Check sheet for the drawn part. Datum: minimum x, y, z corner. Units: mm. A direction names the side the tool comes from. Give positions to 0.01 mm unless a question says otherwise; leave off trailing zeros. Write each loop counter-clockwise with the first axis right and the second up, starting at its lowest first coordinate (ties: lowest second). Pieces come first, ordered by that corner, then holes. Notation, with made-up numbers: (-7, -9.5) - (15, -9.5) arc R24 ccw to (15, 8.5) - close; hole circle Ø3 at (64.25, 38.25). An arc over 180 degrees is marked (long way). Answer as a JSON object with one key per item and string values. Group by question number.
Item 1: Scan lines: line 1 along Y through (x, z) = (26.91, 38); line 2 along X through (y, z) = (26, 38); line 3 along Z through (x, y) = (48, 32). Record each from-to range of solid material in increasing order. Write a range as [from, to].
Item 2: Draft check along X on the marked faces 4, 5, 6 and 7. Enter one of: +X half, -X half, draft (parallel to the pull), parting line (faces both ways), or undercut.
Item 3: Sectioned sample at A-A, the plane y = 26.91. Record the boundary of the cut face in (x, z) (3 decimals), and give its area (3 significant figures).
Item 4: Tool access check on the marked faces 1, 2 and 3. Record the directions out of +Z, -Z, +X, -X, +Y, -Y that give a thin tool (end or side, any length) a straight path to the whole face; none if there is none.
Item 5: Sectioned sample at D-D, the plane y = 5.46. Record the boundary of the cut face in (x, z) (3 decimals), and give its area (3 significant figures).
Item 6: Sectioned sample at C-C, the plane z = 39.5. Record the boundary of the cut face in (x, y), and give its area (3 significant figures).
Item 7: Go/stop test with flat-tipped pins: pin 1 (4.5 mm diameter, centred on x = 26.91, y = 48.36, fed in from -Z); pin 2 (3 mm diameter, centred on y = 28, z = 29, fed in from +X) (3 decimals); pin 3 (7 mm diameter, centred on x = 5.46, y = 26.91, fed in from +Z); pin 4 (8.5 mm diameter, centred on x = 5.46, y = 26.91, fed in from -Z). Record where each tip stops, or that it passes through.
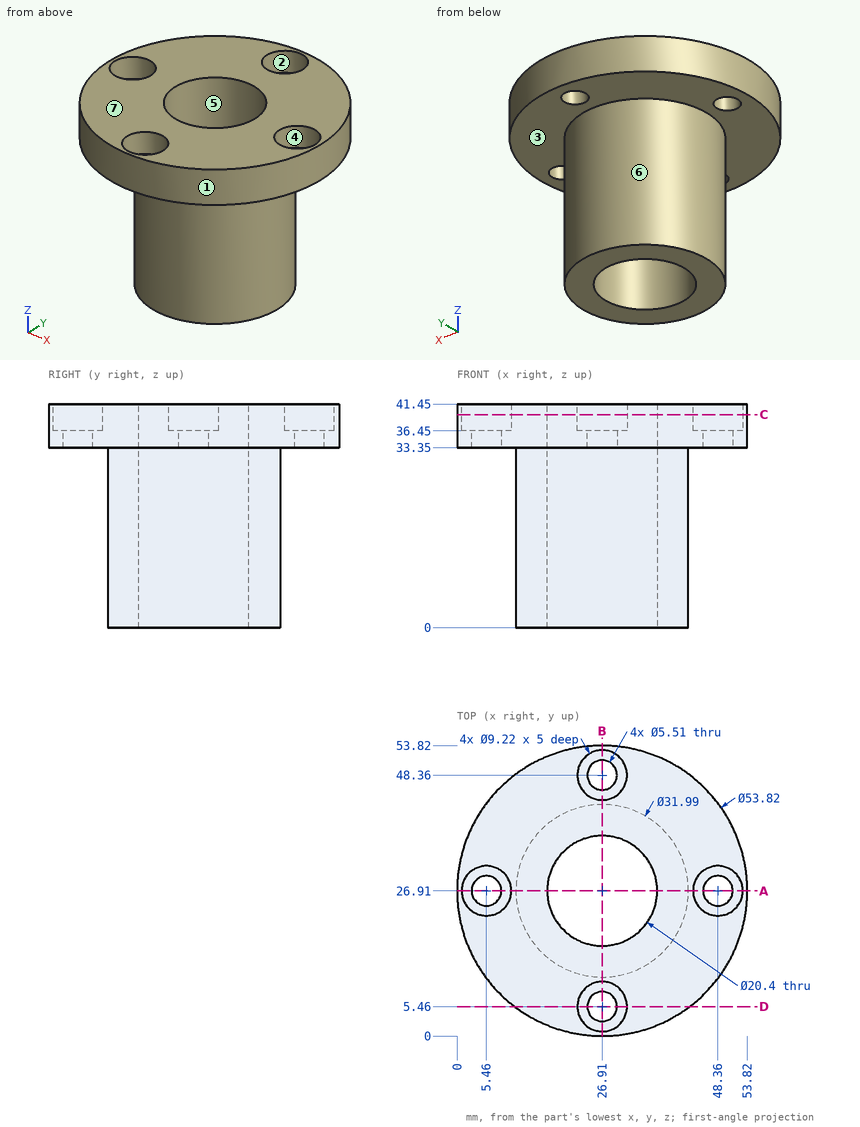
Geometry check:
{
 "1": {"line 1": "[0, 0.85], [10.07, 16.71], [37.11, 43.75], [52.97, 53.82]", "line 2": "[0.02, 0.94], [9.98, 16.75], [37.07, 43.84], [52.88, 53.8]", "line 3": "[33.35, 41.45]"},
 "2": {"face 4": "undercut", "face 5": "undercut", "face 6": "parting line", "face 7": "draft"},
 "3": {"outline": "(0, 33.35) - (2.705, 33.35) - (2.705, 36.45) - (0.85, 36.45) - (0.85, 41.45) - (0, 41.45) - close; (8.215, 33.35) - (10.915, 33.35) - (10.915, 0) - (16.71, 0) - (16.71, 41.45) - (10.07, 41.45) - (10.07, 36.45) - (8.215, 36.45) - close; (37.11, 0) - (42.905, 0) - (42.905, 33.35) - (45.605, 33.35) - (45.605, 36.45) - (43.75, 36.45) - (43.75, 41.45) - (37.11, 41.45) - close; (51.115, 33.35) - (53.82, 33.35) - (53.82, 41.45) - (52.97, 41.45) - (52.97, 36.45) - (51.115, 36.45) - close", "area": "531 mm^2"},
 "4": {"face 1": "+Z, -Z", "face 2": "+Z", "face 3": "-Z"},
 "5": {"outline": "(10.661, 33.35) - (24.155, 33.35) - (24.155, 36.45) - (22.3, 36.45) - (22.3, 41.45) - (10.661, 41.45) - close; (29.665, 33.35) - (43.159, 33.35) - (43.159, 41.45) - (31.52, 41.45) - (31.52, 36.45) - (29.665, 36.45) - close", "area": "200 mm^2"},
 "6": {"outline": "circle Ø53.82 at (26.91, 26.91); hole circle Ø9.22 at (5.46, 26.91); hole circle Ø20.4 at (26.91, 26.91); hole circle Ø9.22 at (26.91, 5.46); hole circle Ø9.22 at (26.91, 48.36); hole circle Ø9.22 at (48.36, 26.91)", "area": "1,680 mm^2"},
 "7": {"pin 1": "through", "pin 2": "x = 42.905", "pin 3": "z = 36.45", "pin 4": "z = 33.35"}
}
